The listing builds one solid part. Answer for the finished solid, in the listing's coordinates (mm). A direction names the side the tool comes from. Round coordinates to 2 decimals unless told otherwise and drop trailing zeros. Write each loop counter-clockwise with the first axis right and the second up, starting at its lowest first coordinate (ties: lowest second). Pieces come first, ordered by that corner, then holes. Notation, with made-up numbers: (9.25, -25.5) - (42.25, -25.5) arc R10 cw to (42.25, -11.5) - close; hole circle Ø10 at (2.5, 34). An arc over 180 degrees is marked (long way). Use a Markdown table: item, result. Add a question column.
1) Find the intervals of material crossed by probe 1 along X at (y, z) = (59, 0); probe 2 along X at (y, z) = (8.5, 0); probe 3 along Y at (x, z) = (-13, 3), in increasing order. Write a range as from..to.
2) Each of these flat-tipped pins is pushed along its axis until it touches: P1, Ø4, axis at x = -25, z = -17, coming from the +Y side; P2, Ø7, axis at x = 0, z = 0, coming from the -Y side; P3, Ø6, axis at y = 64.5, z = -2.5, coming from the +X side; P4, Ø8, axis at y = 78.5, z = -14, coming from the -X side. Where does it stop, or does it pass through?
3) A cutting plane is placed at A-A (y = 17.5). Give the vertices of the cut face in (x, z).
4) Determine the mould class of faces 1 (the flat face through (0, 30, 7)), 2 (the flat face through (0, 88, -7)), 3 (the cylindrical face through (-15.62, 86.48, -3.47)) for opening direction Z: +Z half, -Z half, draft (parallel to the pull), parting line (faces both ways), or undercut.
5) A cutting plane is placed at B-B (y = 47). Give the vertices of the cut face in (x, z), then the cut area to 3 significant figures.
6) A tool of negligible diameter and unlimited length cuts with its end or side. For faces 4 (the cylindrical face through (-20.013, 18.549, -4.444)), 5 (the flat face through (-16.3, 1.5, -0.3)), 6 (the cylindrical face through (-19.524, 76.381, -4.336)), 7 (the cylindrical face through (0, 59, -6)), from which of +Z, -Z, +X, -X, +Y, -Y can it reach the whole face along a straight path? Write none if from no direction.
```python
from build123d import *

# Parameters (mm, degrees)
F2_R = 6


with BuildPart() as f1:
    # F0 (on Right) → F1 (revolve)
    with BuildSketch(Plane.YZ):
        with BuildLine():
            Line((30, 6), (88, 6))
            Line((88, 6), (88, 16))
            Line((88, 16), (85, 16))
            Line((85, 16), (85, 20))
            Line((85, 20), (68, 20))
            Line((68, 20), (68, 32))
            Line((68, 32), (56, 32))
            ThreePointArc((56, 32), (50, 26), (44, 32))
            Line((44, 32), (0, 32))
            Line((0, 32), (0, 25))
            Line((0, 25), (1.5, 25))
            Line((1.5, 25), (1.5, 16))
            Line((1.5, 16), (12, 16))
            Line((12, 16), (12, 12.5))
            Line((12, 12.5), (15, 12.5))
            Line((15, 12.5), (15, 20.5))
            Line((15, 20.5), (22, 20.5))
            Line((22, 20.5), (22, 16))
            Line((22, 16), (30, 16))
            Line((30, 16), (30, 6))
        make_face()
    revolve(axis=Axis((0, 49.247101, 0), (0, 1, 0)))

    # F2
    f2_edges = [f1.edges().sort_by_distance(p)[0] for p in [
        (0, 0, -32),
    ]]
    fillet(f2_edges, radius=F2_R)


solid = f1.part
```
Entries:
| question | item | result |
|---|---|---|
| 1 | probe 1 | x = -32..-6, 6..32 |
| 1 | probe 2 | x = -32..-16, 16..32 |
| 1 | probe 3 | y = 12..15, 30..88 |
| 2 | P1 | stops at y = 68 |
| 2 | P2 | passes through |
| 2 | P3 | stops at x = 32 |
| 2 | P4 | stops at x = -17.32 |
| 3 | outline | circle Ø64 at (0, 0); hole circle Ø41 at (0, 0) |
| 4 | face 1 | undercut |
| 4 | face 2 | draft |
| 4 | face 3 | parting line |
| 5 | outline | circle Ø53.61 at (0, 0); hole circle Ø12 at (0, 0) |
| 5 | area | 2,140 mm² |
| 6 | face 4 | none |
| 6 | face 5 | -Y |
| 6 | face 6 | +Y |
| 6 | face 7 | +Y, -Y |
